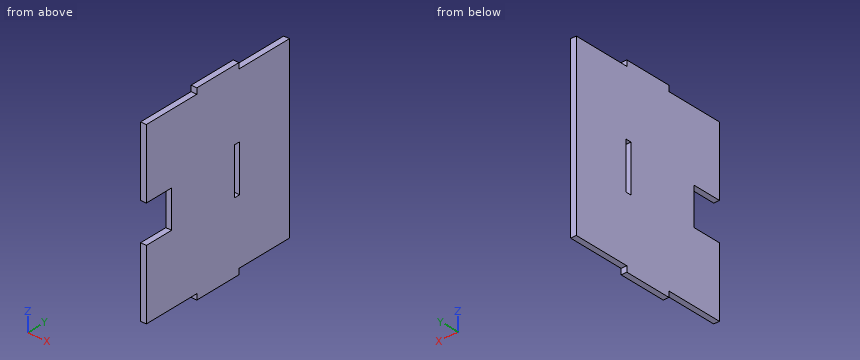
Autodesk Inventor part; units mm, degrees
ref_plane "YZ Plane" through (0, 0, 0) normal (1, 0, 0) x (0, 1, 0)
ref_plane "XZ Plane" through (0, 0, 0) normal (0, 1, 0) x (-1, 0, 0)
ref_plane "XY Plane" through (0, 0, 0) normal (0, 0, 1) x (1, 0, 0)
sketch "Sketch1" plane through (0, 0, 0) normal (1, 0, 0) x (0, 1, 0)
  line L0 (0, -94) -> (30, -94)
  line L1 (30, -94) -> (30, -97)
  line L2 (30, -97) -> (55, -97)
  line L3 (55, -97) -> (55, -94)
  line L4 (55, -94) -> (85, -94)
  line L5 (85, -94) -> (85, 0)
  line L6 (85, 0) -> (55, 0)
  line L7 (55, 0) -> (55, 3)
  line L8 (55, 3) -> (30, 3)
  line L9 (30, 3) -> (30, 0)
  line L10 (30, 0) -> (0, 0)
  line L11 (0, 0) -> (0, -37)
  line L12 (0, -37) -> (15, -37)
  line L13 (15, -37) -> (15, -57)
  line L14 (15, -57) -> (0, -57)
  line L15 (0, -57) -> (0, -94)
  line L16 (0, -47) -> (52.5, -47) construction
  line L17 (52.5, -47) -> (80, -47) construction
  line L18 (0, -47) -> (52.5, -47) construction
  line L19 (52.5, -47) -> (55.5, -47) construction
  line L20 (52.5, -47) -> (52.5, -59.5)
  line L21 (52.5, -59.5) -> (55.5, -59.5)
  line L22 (55.5, -59.5) -> (55.5, -34.5)
  line L23 (55.5, -34.5) -> (52.5, -34.5)
  line L24 (52.5, -34.5) -> (52.5, -47)
  point P0 (42.5, 3)
  dimension "d0" = 94
  dimension "d1" = 30
  dimension "d2" = 3
  dimension "d3" = 25
  dimension "d5" = 30
  dimension "d6" = 94
  dimension "d7" = 30
  dimension "d8" = 3
  dimension "d9" = 25
  dimension "d10" = 3
  dimension "d11" = 30
  dimension "d15" = 15
  dimension "d16" = 20
  dimension "d23" = 27.5
  dimension "d26" = 3
  dimension "d27" = 12.5
  dimension "d28" = 3
  dimension "d29" = 25
  dimension "d30" = 3
  dimension "d31" = 12.5
  dimension "d34" = 52.5
  dimension "d35" = 37
  dimension "d36" = 50
extrude "Extrusion2" add sketch "Sketch1" along normal blind 3
properties part number "Depan"
Source: CAD feature listing. Evaluate the final solid. Frame: model axes, mm. Round coordinates to 2 decimals unless told otherwise and drop trailing zeros. Write each loop counter-clockwise with the first axis right and the second up, starting at its lowest first coordinate (ties: lowest second). Pieces come first, ordered by that corner, then holes. Notation, with made-up numbers: M 32.25,39 L 60.25,39 A12 cw 60.25,53 Z; hole C -31.75,22 d8. An arc over 180 degrees is marked long. Answer as a JSON object with one key per item and string values. Group by question number.
(1) First-contact query: pin 1 (0.9 mm diameter, centred on x = 1, z = -45, fed in from -Y); pin 2 (1.5 mm diameter, centred on x = 1, y = 11, fed in from -Z); pin 3 (0.9 mm diameter, centred on x = 2, y = 10.5, fed in from +Z). Flat tips, straight axial feed; report the tip coordinate or a pass-through.
(2) Section query B-B on x = 0.75. Output: boundary loops of the cut face in (y, z).
(3) Section query C-C on y = 10. Output: boundary loops of the cut face in (x, z).
(4) Section query D-D on y = 58.5. Output: boundary loops of the cut face in (x, z), then the cut area to 3 significant figures.
(5) Ray query, line 1 (Y direction, x = 2.9, z = -51.5); line 2 (Z direction, x = 0.25, y = 54.5); line 3 (Z direction, x = 1.5, y = 57.5). Return the intervals inside material, ascending. Write a range as [from, to].
(6) Section query A-A on z = -41.5. Output: boundary loops of the cut face in (x, y).
Computed values:
{
 "1": {"pin 1": "y = 15", "pin 2": "z = -94", "pin 3": "z = 0"},
 "2": {"outline": "M 0,-94 L 30,-94 L 30,-97 L 55,-97 L 55,-94 L 85,-94 L 85,0 L 55,0 L 55,3 L 30,3 L 30,0 L 0,0 L 0,-37 L 15,-37 L 15,-57 L 0,-57 Z; hole M 52.5,-59.5 L 55.5,-59.5 L 55.5,-34.5 L 52.5,-34.5 Z"},
 "3": {"outline": "M 0,-94 L 3,-94 L 3,-57 L 0,-57 Z; M 0,-37 L 3,-37 L 3,0 L 0,0 Z"},
 "4": {"outline": "M 0,-94 L 3,-94 L 3,0 L 0,0 Z", "area": "282 mm^2"},
 "5": {"line 1": "[15, 52.5], [55.5, 85]", "line 2": "[-97, -59.5], [-34.5, 3]", "line 3": "[-94, 0]"},
 "6": {"outline": "M 0,15 L 3,15 L 3,52.5 L 0,52.5 Z; M 0,55.5 L 3,55.5 L 3,85 L 0,85 Z"}
}
